Autodesk Inventor part; units mm, degrees
ref_plane "YZ Plane" through (0, 0, 0) normal (1, 0, 0) x (0, 1, 0)
ref_plane "XZ Plane" through (0, 0, 0) normal (0, 1, 0) x (-1, 0, 0)
ref_plane "XY Plane" through (0, 0, 0) normal (0, 0, 1) x (1, 0, 0)
sketch "Sketch1" plane through (0, 0, 0) normal (0, 1, 0) x (-1, 0, 0)
  line L0 (-200, 200) -> (200, 200)
  line L1 (200, 200) -> (200, -200)
  line L2 (200, -200) -> (-200, -200)
  line L3 (-200, -200) -> (-200, 200)
  line L4 (-200, 200) -> (200, -200) construction
  line L5 (200, 200) -> (-200, -200) construction
  point P0 (0, 0)
  dimension "d0" = 400
extrude "Extrusion1" add sketch "Sketch1" along normal mid plane 3
sketch "Sketch2" plane through (0, -1.5, 0) normal (0, -1, 0) x (1, 0, 0)
  line L0 (-200, -200) -> (200, -200)
  point P0 (0, 0)
  point P1 (-182, -183)
  point P2 (0, -183)
  point P3 (182, -183)
  dimension "d3" = 182
  dimension "d4" = 182
  dimension "d5" = 17
hole "Hole1" at (-182, -1.5, -183) at (0, -1.5, -183) at (182, -1.5, -183) direction (0, 1, 0) diameter 6 depth 14.2 tip angle 118
sketch "Sketch3" plane through (0, -1.5, 0) normal (0, -1, 0) x (1, 0, 0)
  line L0 (200, 200) -> (-200, 200)
  line L1 (-200, 200) -> (-200, -200)
  point P0 (0, 0)
  point P1 (-186, 100)
  point P2 (-186, 0)
  point P3 (-186, -100)
  dimension "d13" = 100
  dimension "d14" = 100
  dimension "d15" = 100
  dimension "d16" = 14
hole "Hole2" at (-186, -1.5, 100) at (-186, -1.5, 0) at (-186, -1.5, -100) direction (0, 1, 0) diameter 6 depth 14.2 tip angle 118
mirror "Mirror1" about plane through (0, 0, 0) normal (1, 0, 0) of "Hole2"
sketch "Sketch4" plane through (0, 1.5, 0) normal (0, 1, 0) x (1, 0, 0)
  circle A0 centre (-50, 120) radius 9
  line L0 (200, 200) -> (-200, 200)
  line L1 (-200, 200) -> (-200, -200)
  point P0 (0, 0)
  dimension "d24" = 80
  dimension "d25" = 18
  dimension "d26" = 150
extrude "Extrusion2" cut sketch "Sketch4" against normal blind 10
properties part number "HCMUTE-CDT23-KXL_A02" material "PMMA Plastic"
The listing builds one solid part. Answer for the finished solid, in the listing's coordinates (mm). Round coordinates to 2 decimals unless told otherwise and drop trailing zeros. Write each loop counter-clockwise with the first axis right and the second up, starting at its lowest first coordinate (ties: lowest second). Pieces come first, ordered by that corner, then holes. Notation, with made-up numbers: M 52.25,53.25 L 56.25,53.25 A30 ccw 56.25,78.25 Z; hole C -32.75,9 d6. An arc over 180 degrees is marked long. Write each question's results on one line, items separated by ' | '. Start each with the question number.
(1) Find the intervals of material crossed by line 1 (Z direction, x = -186, y = 0.1); line 2 (X direction, y = 0.2, z = 100); line 3 (X direction, y = -0.6, z = -183), in increasing order.
(2) The part is cut by section A-A, the plane x = -50. Write down the section's boundary in (y, z).
(3) Each of these flat-tipped pins is pushed along its axis until it touches: P1, Ø7, axis at x = 0, z = -183, coming from the -Y side; P2, Ø3.5, axis at x = -182, z = -183, coming from the +Y side. Where does it stop, or does it pass through?
(4) Determine the mould class of faces 1 (the cylindrical face through (-59, 0, -120)), 2 (the flat face through (3, -1.5, 3)) for opening direction X: +X half, -X half, draft (parallel to the pull), parting line (faces both ways), or undercut.
(5) The part is cut by section B-B, the plane z = -120. Write down the section's boundary in (x, y).
Worked answers:
1) line 1: z = -200 to -103, -97 to -3, 3 to 97, 103 to 200 | line 2: x = -200 to -189, -183 to 183, 189 to 200 | line 3: x = -200 to -185, -179 to -3, 3 to 179, 185 to 200
2) outline: M -1.5,-200 L 1.5,-200 L 1.5,-129 L -1.5,-129 Z; M -1.5,-111 L 1.5,-111 L 1.5,200 L -1.5,200 Z
3) P1: stops at y = -1.5 | P2: passes through
4) face 1: undercut | face 2: draft
5) outline: M -200,-1.5 L -59,-1.5 L -59,1.5 L -200,1.5 Z; M -41,-1.5 L 200,-1.5 L 200,1.5 L -41,1.5 Z
